Design review of the part built by this model. Coordinates are the model's own, in mm. A direction names the side the tool comes from. Coordinates: 2 decimals unless noted, no trailing zeros. Write each loop counter-clockwise with the first axis right and the second up, starting at its lowest first coordinate (ties: lowest second). Pieces come first, ordered by that corner, then holes.
Q1. Add section B-B, the plane z = 0. Give the boundary of the cut face in (x, y), plus the area to 3 significant figures.
Q2. The part is to be moulded in two halves that separate along Y. For faces 1 (the face through (0, -30, 0)), 2 (the face through (-9, 20, 9)), 3 (the face through (-24.54, -16.69, -24.5)), say which applies: +Y half, -Y half, draft (parallel to the pull), parting line (faces both ways), or undercut.
Q3. Machinability: for faces 4 (the face through (25.4, -16, 0)), 5 (the face through (-8.618, 22.479, 20.784)), 6 (the face through (10, 0, 10)), which of the approach directions +Z, -Z, +X, -X, +Y, -Y give a long, thin tool a straight path to every point of the face, cutting with its end or side? Answer none if there is none.
Q4. Clearance check with flat-ended pins moving along their axes: pin 1 Ø2 at (x, y) = (-7.5, 6) entering from +Z; pin 2 Ø3 at (x, y) = (10, 12.5) entering from -Z; pin 3 Ø5 at (x, y) = (-4.5, 12) entering from +Z. State where each tip first meets the part, or that it passes through.
Q5. Add section A-A, the plane x = 0. Give the boundary of the cut face in (y, z).
Q6. To check wall thickness, follow probe 1 along Y at (x, z) = (10, -18); probe 2 along Y at (x, z) = (-19.5, 22.5); probe 3 along Z at (x, y) = (-2.5, 10.5). State the ranges of each line that lie inside material, in increasing order.
from build123d import *

# Parameters (mm, degrees)
SKETCH1_W           = 50.8
SKETCH1_H           = 50.8
BOSS_EXTRUDE1_DEPTH = 30
SKETCH2_R           = 12.5
BOSS_EXTRUDE2_DEPTH = 20
BOSS_EXTRUDE3_START = 20
SKETCH3_R           = 22.5
BOSS_EXTRUDE3_DEPTH = 5
FILLET1_R           = 3
FILLET2_R           = 1


with BuildPart() as part:
    # Sketch1 → Boss-Extrude1 (new body)
    with BuildSketch(Plane(origin=(0, 0, 0), x_dir=(1, 0, 0), z_dir=(0, 1, 0))):
        Rectangle(SKETCH1_W, SKETCH1_H)
    extrude(amount=-BOSS_EXTRUDE1_DEPTH)

    # Sketch2 → Boss-Extrude2 (add)
    with BuildSketch(Plane(origin=(0, 0, 0), x_dir=(1, 0, 0), z_dir=(0, 1, 0))):
        with Locations(Location((0, 0, 0), (0, 0, 270))):
            Circle(SKETCH2_R)
    extrude(amount=BOSS_EXTRUDE2_DEPTH)

    # Sketch3 → Boss-Extrude3 (add)
    with BuildSketch(Plane(origin=(0, 0, 0), x_dir=(1, 0, 0), z_dir=(0, 1, 0)).offset(BOSS_EXTRUDE3_START)):
        with Locations(Location((0, 0, 0), (0, 0, 270))):
            Circle(SKETCH3_R)
    extrude(amount=BOSS_EXTRUDE3_DEPTH)

    # Fillet1
    fillet1_edges = [part.edges().sort_by_distance(p)[0] for p in [
        (0, 0, 25.4),
        (-25.4, 0, 0),
        (0, 0, -25.4),
        (25.4, 0, 0),
        (25.4, -15, 25.4),
        (-25.4, -15, 25.4),
        (-25.4, -15, -25.4),
        (25.4, -15, -25.4),
    ]]
    fillet(fillet1_edges, radius=FILLET1_R)

    # Fillet2
    fillet2_edges = [part.edges().sort_by_distance(p)[0] for p in [
        (0, 20, -22.5),
        (0, 25, -22.5),
    ]]
    fillet(fillet2_edges, radius=FILLET2_R)


solid = part.part
Here are the results:
1. outline: (-25.4, -30) - (25.4, -30) - (25.4, -3) arc R3 ccw to (22.4, 0) - (12.5, 0) - (12.5, 20) - (21.5, 20) arc R1 ccw to (22.5, 21) - (22.5, 24) arc R1 ccw to (21.5, 25) - (-21.5, 25) arc R1 ccw to (-22.5, 24) - (-22.5, 21) arc R1 ccw to (-21.5, 20) - (-12.5, 20) - (-12.5, 0) - (-22.4, 0) arc R3 ccw to (-25.4, -3) - close
1. area: 2,240 mm2
2. face 1: -Y half
2. face 2: undercut
2. face 3: draft
3. face 4: +Z, -Z, +X, +Y, -Y
3. face 5: +Y
3. face 6: none
4. pin 1: stops at z = 10.68
4. pin 2: stops at z = -9.17
4. pin 3: stops at z = 12.34
5. outline: (-30, -25.4) - (-3, -25.4) arc R3 ccw to (0, -22.4) - (0, -12.5) - (20, -12.5) - (20, -21.5) arc R1 ccw to (21, -22.5) - (24, -22.5) arc R1 ccw to (25, -21.5) - (25, 21.5) arc R1 ccw to (24, 22.5) - (21, 22.5) arc R1 ccw to (20, 21.5) - (20, 12.5) - (0, 12.5) - (0, 22.4) arc R3 ccw to (-3, 25.4) - (-30, 25.4) - close
6. probe 1: y = -30 to 0, 20 to 25
6. probe 2: y = -30 to 0
6. probe 3: z = -12.25 to 12.25
